Here's how the part is built. I have some questions about the finished solid (model axes, mm). A direction names the side the tool comes from. Round coordinates to 2 decimals unless told otherwise and drop trailing zeros. Write each loop counter-clockwise with the first axis right and the second up, starting at its lowest first coordinate (ties: lowest second). Pieces come first, ordered by that corner, then holes. Notation, with made-up numbers: (79, 72.25) - (126, 72.25) arc R25 ccw to (126, 86.25) - close; hole circle Ø2 at (71, 60). An arc over 180 degrees is marked (long way). One line per question, with ' | ' between items. Start each with the question number.
(1) Imagine slicing it at C-C (y = 125). Write out the boundary of the cut face in (x, z), plus the area to 3 significant figures.
(2) Will these pins go through, and if not, where does the flat tip stop? pin 1 (1 mm diameter, centred on x = 21.5, z = -3, fed in from +Y); pin 2 (1 mm diameter, centred on x = 109, z = -2, fed in from +Y); pin 3 (1.5 mm diameter, centred on x = 29.5, z = -1, fed in from +Y).
(3) Imagine slicing it at B-B (x = 0). Write out the boundary of the cut face in (y, z).
(4) Imagine slicing it at A-A (z = -3.95). Write out the boundary of the cut face in (x, y), plus the area to 3 significant figures.
(5) If I drill on L1, parallel to Y at x = 119, z = -3.85; L2, parallel to Y at x = 52.5, z = -1.15; L3, parallel to X at y = 140, z = -4, over which ranges is the centre line in solid material (lowest first)?
(6) For faces 1 (the flat face through (59.85, 93.63, -2.5)), 2 (the flat face through (59.816, 97.671, -2.504)), which set-ups out of +Z, -Z, +X, -X, +Y, -Y let a thin tool reach every point of the face, with its end or its side?
(7) Thinking about a two-plate mould opening in X: for faces 3 (the flat face through (63, 58, -5.08)), 4 (the flat face through (81.7, 80.3, -2.5)), 5 (the cylindrical face through (-7.309, -8.788, -2.504)), which applies, pulls with the +X half, pulls with the -X half, needs draft (parallel to the pull), parting line crosses it, or undercut?
Autodesk Inventor part; units mm, degrees
ref_plane "YZ Plane" through (0, 0, 0) normal (1, 0, 0) x (0, 1, 0)
ref_plane "XZ Plane" through (0, 0, 0) normal (0, 1, 0) x (-1, 0, 0)
ref_plane "XY Plane" through (0, 0, 0) normal (0, 0, 1) x (1, 0, 0)
sketch "Sketch1" plane through (0, 0, 0) normal (0, 0, 1) x (1, 0, 0)
  arc A0 (-8.9464, 7.1138) -> (8.9464, -7.1138) centre (0, 0) ccw
  arc A1 (148.494, 168.382) -> (130.6012, 182.6097) centre (139.5476, 175.4959) ccw
  line L0 (-8.9464, 7.1138) -> (130.6012, 182.6097)
  line L1 (148.494, 168.382) -> (8.9464, -7.1138)
  arc A2 (-10.9345, 8.6947) -> (10.9345, -8.6947) centre (0, 0) ccw
  arc A3 (150.4821, 166.8012) -> (128.6131, 184.1906) centre (139.5476, 175.4959) ccw
  line L2 (128.6131, 184.1906) -> (-10.9345, 8.6947)
  line L3 (150.4821, 166.8012) -> (10.9345, -8.6947)
  dimension "d0" = 22.86
  dimension "d1" = 22.86
  dimension "d3" = 27.94
  dimension "d4" = 27.94
extrude "Extrusion1" add sketch "Sketch1" against normal blind 5.08
properties part number "Lift down banding"
Check sheet entries:
1) outline: (81.55, -5.08) - (84.79, -5.08) - (84.79, 0) - (81.55, 0) - close; (114, -5.08) - (117.24, -5.08) - (117.24, 0) - (114, 0) - close | area: 33.0 mm^2
2) pin 1: y = 50.11 | pin 2: y = 160.15 | pin 3: y = 60.49
3) outline: (-13.97, -5.08) - (-11.43, -5.08) - (-11.43, 0) - (-13.97, 0) - close; (18.36, -5.08) - (22.45, -5.08) - (22.45, 0) - (18.36, 0) - close
4) outline: (-10.93, 8.69) arc R13.97 ccw to (10.93, -8.69) - (150.48, 166.8) arc R13.97 ccw to (128.61, 184.19) - close; hole (-8.95, 7.11) arc R11.43 ccw to (8.95, -7.11) - (148.49, 168.38) arc R11.43 ccw to (130.6, 182.61) - close | area: 1,340 mm^2
5) L1: 127.21 to 131.29, 168.02 to 172.1 | L2: 43.58 to 47.66, 84.39 to 88.47 | L3: 93.47 to 96.72, 125.93 to 129.17
6) face 1: +Z, -Z | face 2: +Z, -Z, -X, +Y
7) face 3: needs draft | face 4: pulls with the +X half | face 5: undercut
